from build123d import *

# Parameters (mm, degrees)
F0_R            = 101.6
F0_R_2          = 14.2875
F1_DEPTH        = 3.175
F2_R            = 2.4892
F3_DEPTH        = 3.176
F3_COPIES_COUNT = 6
F4_R            = 2.3622
F5_DEPTH        = 3.176


# Not quite as in the source:
# - a pattern or mirror of a feature is missing from the dataset's text; its kind, count and spacing are read off the source's solid


with BuildPart() as f1:
    # F0 (on Top) → F1 (new body)
    with BuildSketch(Plane.XY):
        Circle(F0_R)
        Circle(F0_R_2, mode=Mode.SUBTRACT)
    extrude(amount=F1_DEPTH)

    # F2 (on face) → F3 (cut, through all)
    with BuildSketch(Plane.XY.offset(3.175)):
        with Locations((0, 23.8125)):
            Circle(F2_R)
        with Locations((0, 76.2)):
            Circle(F2_R)
        with Locations((25.4, 43.9940905122)):
            Circle(F2_R)
    f3 = extrude(amount=-F3_DEPTH, mode=Mode.SUBTRACT)

    # F3_copies: F3 ×6 about axis
    f3_copies_axis = Axis((0, 0, 0), (0, 0, 1))
    for i in range(1, F3_COPIES_COUNT):
        add(f3.rotate(f3_copies_axis, i * 360 / F3_COPIES_COUNT), mode=Mode.SUBTRACT)

    # F4 (on face) → F5 (cut, through all)
    with BuildSketch(Plane.XY.offset(3.175)):
        with Locations((0, 40.2743678674)):
            Circle(F4_R)
        with Locations((38.3032, 12.4454641087)):
            Circle(F4_R)
        with Locations((23.6726794779, -32.5826480425)):
            Circle(F4_R)
        with Locations((-23.6726794779, -32.5826480425)):
            Circle(F4_R)
        with Locations((-38.3032, 12.4454641087)):
            Circle(F4_R)
    extrude(amount=-F5_DEPTH, mode=Mode.SUBTRACT)


solid = f1.part
Verification items for the finished model (mm, model axes). Round coordinates to 2 decimals unless told otherwise and drop trailing zeros. Write each loop counter-clockwise with the first axis right and the second up, starting at its lowest first coordinate (ties: lowest second). Pieces come first, ordered by that corner, then holes.
(1) Depth check by flat-ended pin: pin 1 Ø4 at (x, y) = (65.99, 38.1) entering from +Z; pin 2 Ø1 at (x, z) = (-7, 0.5) entering from -Y; pin 3 Ø1 at (y, z) = (15.5, 3) entering from -X. Enter the tip coordinate at first touch or a pass-through.
Returned:
pin 1: passes through
pin 2: stops at y = -101.39
pin 3: stops at x = -100.49
(2) Material ranges on line 1 (X direction, y = -9, z = 0.45); line 2 (X direction, y = 25, z = 1); line 3 (X direction, y = -60.5, z = 2.3), recorded low to high.
Returned:
line 1: x = -101.2 to -11.1, 11.1 to 101.2
line 2: x = -98.48 to -2.19, 2.19 to 98.48
line 3: x = -81.62 to 81.62
(3) Section check D-D (y = -51). Enter the section's corners in (x, z) (3 decimals), plus the area to 3 significant figures.
Returned:
outline: (-87.872, 0) - (87.872, 0) - (87.872, 3.175) - (-87.872, 3.175) - close
area: 558 mm2
(4) Section check C-C (x = 58). Enter the section's corners in (y, z) (3 decimals).
Returned:
outline: (-83.418, 0) - (83.418, 0) - (83.418, 3.175) - (-83.418, 3.175) - close
(5) Section check B-B (z = 0.6). Give the number of separate pieces and of enclosed holes in the cut face, plus the area to 4 significant figures.
Returned:
separate pieces: 1
enclosed holes: 24
area: 31,350 mm2
(6) Section check A-A (y = -76.2). Enter the section's corners in (x, z) (3 decimals).
Returned:
outline: (-67.202, 0) - (-2.489, 0) - (-2.489, 3.175) - (-67.202, 3.175) - close; (2.489, 0) - (67.202, 0) - (67.202, 3.175) - (2.489, 3.175) - close
(7) Mould release check, pull along X, two halves, no side actions. Record for faces 1 (the cylindrical face through (-63.617, -37.352, 1.61)), 2 (the cylindrical face through (40.485, 11.541, 1.61)), 3 (the flat face through (21, 1, 3.175)), 4 (the cylindrical face through (-22.025, -99.184, 1.565)): pulls with the +X half, pulls with the -X half, needs draft (parallel to the pull), parting line crosses it, or undercut.
Returned:
face 1: undercut
face 2: undercut
face 3: needs draft
face 4: parting line crosses it
